from build123d import *

# Parameters (mm, degrees)
F0_W     = 76.2
F0_H     = 199.9996
F1_DEPTH = 4.499991
F2_R     = 19.05
F3_DEPTH = 120
F4_R     = 19
F5_DEPTH = 690
F6_W     = 688.959937
F6_H     = 36.997854
F7_DEPTH = 178


with BuildPart() as f1:
    # F0 (on Front) → F1 (new body, symmetric)
    with BuildSketch(Plane.XZ):
        Rectangle(F0_W, F0_H)
    extrude(amount=F1_DEPTH, both=True)

    # F2 (on face) → F3 (join)
    with BuildSketch(Plane.XZ.offset(4.499991)):
        with Locations((0, -80.9498)):
            Circle(F2_R)
    extrude(amount=F3_DEPTH)

    # F4 (on face) → F5 (join)
    with BuildSketch(Plane(origin=(0, 4.499991, 0), x_dir=(-1, 0, 0), z_dir=(0, 1, 0))):
        with Locations((0, 80.9998)):
            Circle(F4_R)
    extrude(amount=F5_DEPTH)

    # F6 (on Right) → F7 (join)
    with BuildSketch(Plane.YZ):
        with Locations((349.496255, 80.745302)):
            Rectangle(F6_W, F6_H)
    extrude(amount=F7_DEPTH)


solid = f1.part
CAD build for the part. Positions are in the model's coordinates, mm. A direction names the side the tool comes from. Give positions to 0.01 mm unless a question says otherwise; leave off trailing zeros. Write each loop counter-clockwise with the first axis right and the second up, starting at its lowest first coordinate (ties: lowest second). Pieces come first, ordered by that corner, then holes. Notation, with made-up numbers: M -23.5,-15 L -12.5,-15 A32 cw -12.5,13 Z; hole C 31,66 d10. An arc over 180 degrees is marked long. Put each result on its own line as item: value. Start each with the question number.
(1) Flat gauge pins, fed straight in: pin 1 Ø7 at (y, z) = (0, 18) entering from +X; pin 2 Ø2 at (x, y) = (-11, 474.5) entering from +Z; pin 3 Ø11 at (x, z) = (101.5, 81.5) entering from +Y. Where does each tip first touch, or does it go through?
(2) Which spindle directions (+Z, -Z, +X, -X, +Y, -Y) get a long thin tool onto all of the face, cutting with end or side? Do faces 1 (the face through (-4.13, -63.66, -99.547)), 2 (the face through (90, 345, 99.244)). Say none if no direction does.
(3) Band-saw the part on B-B, the plane x = -7.5. Write the cut outline in (y, z).
(4) Band-saw the part on A-A, the plane z = -19.5. Write the cut outline in (x, y), and give its area (3 significant figures).
(5) Band-saw the part on C-C, the plane y = 246.5. Write the cut outline in (x, z), and give its area (3 significant figures).
(6) Probe L1, parallel to Z at x = 166, y = 589; L2, parallel to X at y = 536, z = 78.5; L3, parallel to Y at x = 16, z = 85.5. List the from-to ranges inside material, lowest first.
Response values:
1. pin 1: stops at x = 38.1
1. pin 2: stops at z = 97.16
1. pin 3: stops at y = 693.98
2. face 1: -Y
2. face 2: +Z, +X, +Y
3. outline: M -124.5,-98.46 L -4.5,-98.46 L -4.5,-100 L 4.5,-100 L 4.5,63.54 L 694.5,63.54 L 694.5,98.46 L 4.5,98.46 L 4.5,100 L -4.5,100 L -4.5,-63.44 L -124.5,-63.44 Z
4. outline: M -38.1,-4.5 L 38.1,-4.5 L 38.1,4.5 L -38.1,4.5 Z
4. area: 686 mm2
5. outline: M 3.05,62.25 L 178,62.25 L 178,99.24 L 5.3,99.24 A19 ccw long Z
5. area: 7,160 mm2
6. L1: z = 62.25 to 99.24
6. L2: x = -18.83 to 178
6. L3: y = -4.5 to 694.5
